The figure shows three views and two pictorial views of one solid part (mm, origin at its lowest corner). Answer the questions. A direction names the side the tool comes from. Give positions to 0.01 mm unless a question says otherwise; leave off trailing zeros. Order: outer loops, then holes, each group sorted by start corner. A loop starts at its lowest first (then second) coordinate and runs counter-clockwise, first axis right, second up. Notation, with made-up numbers: (47.25, -18.5) - (66.25, -18.5) arc R28 cw to (66.25, 17.5) - close; hole circle Ø10 at (-22.5, -10.5). An arc over 180 degrees is marked (long way). Answer as a JSON object with one key per item and string values. Group by question number.
Q1. Consider line 1 (Z direction, x = 10, y = 8.35); line 2 (Y direction, x = 19, z = 16); line 3 (X direction, y = 7, z = 6). Determine where each line is inside the solid, lowest interval first.
Q2. A cutting plane is placed at D-D, the plane x = 24. Give the vertices of the cut face in (y, z).
Q3. A cutting plane is placed at B-B, the plane z = 25. Give the vertices of the cut face in (x, y).
Q4. For the marked faces 1, 2, 3 and 4, determine the directions among +Z, -Z, +X, -X, +Y, -Y from which every point of the face is accessible in a straight line to the end or side of a thin tool.
Q5. Given pin 1 (10 mm diameter, centred on x = 23, z = 25.5, fed in from -Y); pin 2 (1 mm diameter, centred on y = 6, z = 5.5, fed in from -X); pin 3 (1.2 mm diameter, centred on x = 18.5, y = 2.5, fed in from -Z); pin 4 (1.5 mm diameter, centred on y = 1.5, z = 25, fed in from +X), each flat-ended and moving along its own axis, determine where each tip first touches the part or whether it passes through.
Q6. The mould has two halves that part along X. Classify the marked faces 5, 6 and 7: released by +X, released by -X, zero draft, split by the parting line, or undercut.
Q7. A cutting plane is placed at A-A, the plane y = 6.5. Give the vertices of the cut face in (x, z).
Q8. A cutting plane is placed at C-C, the plane x = 10. Give the vertices of the cut face in (y, z).
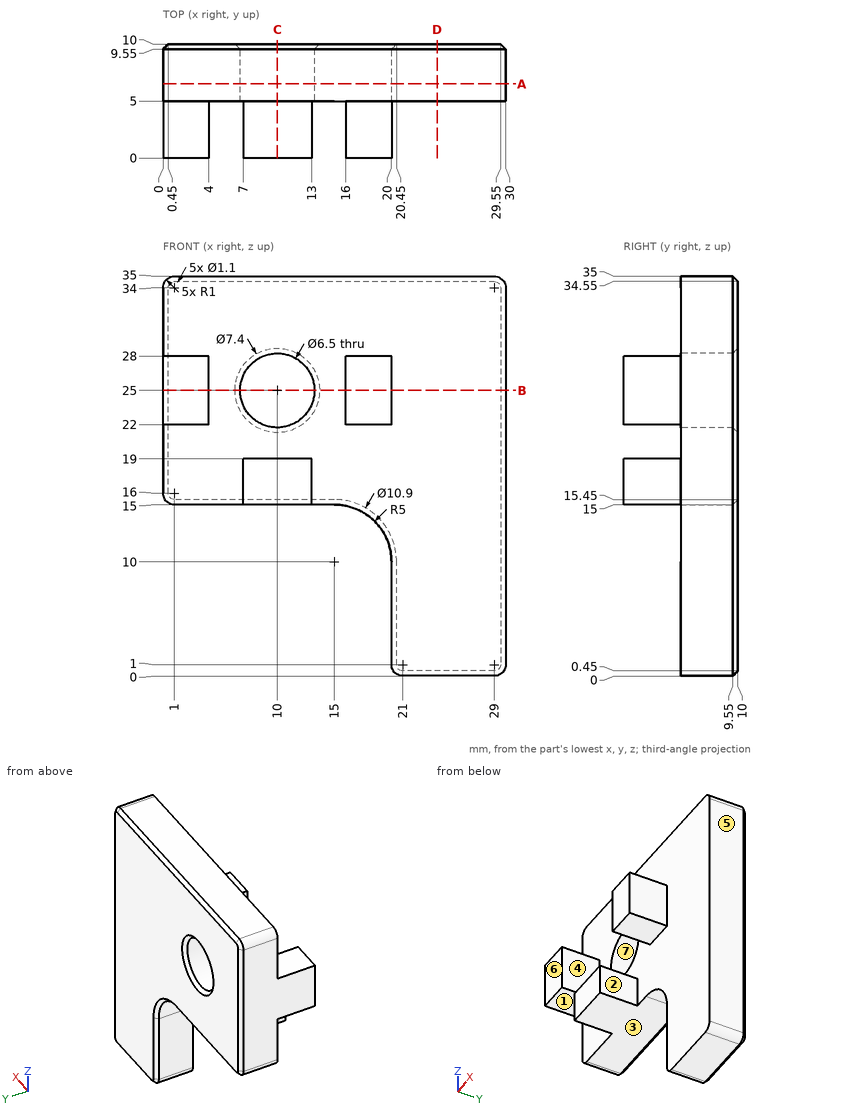
Reply:
{
 "1": {"line 1": "z = 15 to 21.75, 28.25 to 35", "line 2": "y = 5 to 10", "line 3": "x = 20 to 30"},
 "2": {"outline": "(5, 0) - (9.55, 0) - (10, 0.45) - (10, 34.55) - (9.55, 35) - (5, 35) - close"},
 "3": {"outline": "(0, 0) - (4, 0) - (4, 5) - (6.75, 5) - (6.75, 9.55) - (6.3, 10) - (0.45, 10) - (0, 9.55) - close; (13.25, 5) - (16, 5) - (16, 0) - (20, 0) - (20, 5) - (30, 5) - (30, 9.55) - (29.55, 10) - (13.7, 10) - (13.25, 9.55) - close"},
 "4": {"face 1": "-Z, +X, -X, -Y", "face 2": "+Z, -Z, +X, -Y", "face 3": "-Z, -X, +Y, -Y", "face 4": "+Z, -Z, -Y"},
 "5": {"pin 1": "stops at y = 0", "pin 2": "stops at x = 20", "pin 3": "stops at z = 22", "pin 4": "stops at x = 20"},
 "6": {"face 5": "released by +X", "face 6": "zero draft", "face 7": "undercut"},
 "7": {"outline": "(0, 16) arc R1 ccw to (1, 15) - (15, 15) arc R5 cw to (20, 10) - (20, 1) arc R1 ccw to (21, 0) - (29, 0) arc R1 ccw to (30, 1) - (30, 34) arc R1 ccw to (29, 35) - (1, 35) arc R1 ccw to (0, 34) - close; hole circle Ø6.5 at (10, 25)"},
 "8": {"outline": "(0, 15) - (9.55, 15) - (10, 15.45) - (10, 21.3) - (9.55, 21.75) - (5, 21.75) - (5, 19) - (0, 19) - close; (5, 28.25) - (9.55, 28.25) - (10, 28.7) - (10, 34.55) - (9.55, 35) - (5, 35) - close"}
}
